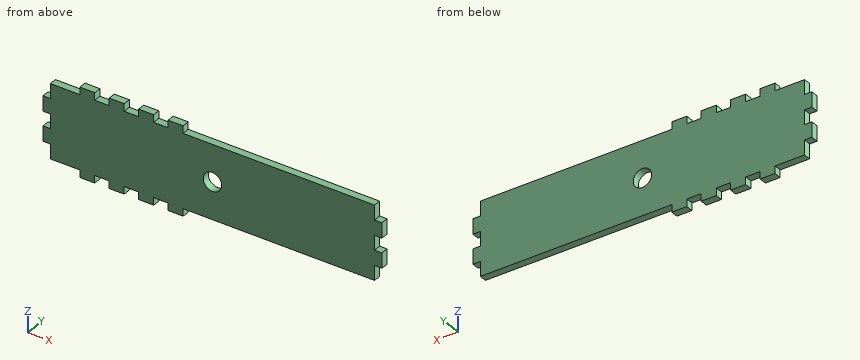
```python
from build123d import *

# Parameters (mm, degrees)
SKETCH1_R           = 7.9375
BOSS_EXTRUDE1_DEPTH = 6.35


with BuildPart() as part:
    # Sketch1 → Boss-Extrude1 (new body)
    with BuildSketch(Plane(origin=(0, 0, 0), x_dir=(1, 0, 0), z_dir=(0, 1, 0))):
        Polygon((279.4, 0), (279.4, -12.573), (285.75, -12.573), (285.75, -25.527), (279.4, -25.527), (279.4, -37.973), (285.75, -37.973), (285.75, -50.927), (279.4, -50.927), (279.4, -63.5), (114.427, -63.5), (114.427, -69.85), (101.473, -69.85), (101.473, -63.5), (89.027, -63.5), (89.027, -69.85), (76.073, -69.85), (76.073, -63.5), (63.627, -63.5), (63.627, -69.85), (50.673, -69.85), (50.673, -63.5), (38.227, -63.5), (38.227, -69.85), (25.4, -69.85), (25.4, -63.5), (0, -63.5), (0, -50.927), (-6.35, -50.927), (-6.35, -37.973), (0, -37.973), (0, -25.527), (-6.35, -25.527), (-6.35, -12.573), (0, -12.573), (0, 0), (25.4, 0), (25.4, 6.35), (38.227, 6.35), (38.227, 0), (50.673, 0), (50.673, 6.35), (63.627, 6.35), (63.627, 0), (76.073, 0), (76.073, 6.35), (89.027, 6.35), (89.027, 0), (101.473, 0), (101.473, 6.35), (114.427, 6.35), (114.427, 0), align=None)
        with Locations((139.7, -31.75)):
            Circle(SKETCH1_R, mode=Mode.SUBTRACT)
    extrude(amount=BOSS_EXTRUDE1_DEPTH)


solid = part.part
```
For this review, take the finished solid that the model builds, in its own axes (mm). Give positions to 0.01 mm unless a question says otherwise; leave off trailing zeros. Write each loop counter-clockwise with the first axis right and the second up, starting at its lowest first coordinate (ties: lowest second). Pieces come first, ordered by that corner, then holes. Notation, with made-up numbers: M 84.5,63.25 L 97.5,63.25 A20 cw 97.5,83.25 Z; hole C 8.5,81.25 d7. An arc over 180 degrees is marked long. One line per item, written item: value.
1) For P1, Ø1.5, axis at x = 234, y = 4, coming from the +Z side; P2, Ø3, axis at x = 92, y = 4, coming from the -Z side; P3, Ø3, axis at y = 2, z = 32, coming from the -X side, all flat-tipped, find the tip position at first contact; note any pin that passes through.
Results are:
P1: stops at z = 63.5
P2: stops at z = 0
P3: stops at x = 0
2) Take a section at B-B, the plane z = 31.75. Write out the cut boundary in (x, y), then the cut area to 3 significant figures.
Results are:
outline: M 0,0 L 131.76,0 L 131.76,6.35 L 0,6.35 Z; M 147.64,0 L 279.4,0 L 279.4,6.35 L 147.64,6.35 Z
area: 1,670 mm²
3) Take a section at A-A, the plane x = 139.7. Write out the cut boundary in (y, z).
Results are:
outline: M 0,0 L 6.35,0 L 6.35,23.81 L 0,23.81 Z; M 0,39.69 L 6.35,39.69 L 6.35,63.5 L 0,63.5 Z
4) Take a section at C-C, the plane x = 241. Write out the cut boundary in (y, z), then the cut area to 3 significant figures.
Results are:
outline: M 0,0 L 6.35,0 L 6.35,63.5 L 0,63.5 Z
area: 403 mm²
5) For line 1 (X direction, y = 2.5, z = -1.5); line 2 (X direction, y = 5, z = 32); line 3 (Z direction, x = 139.7, y = 3.25), list the stretches that pass through material, from the lowest coordinate up. Write a range as from..to.
Results are:
line 1: x = 25.4..38.23, 50.67..63.63, 76.07..89.03, 101.47..114.43
line 2: x = 0..131.77, 147.63..279.4
line 3: z = 0..23.81, 39.69..63.5
